Autodesk Inventor part; units mm, degrees
ref_plane "YZ Plane" through (0, 0, 0) normal (1, 0, 0) x (0, 1, 0)
ref_plane "XZ Plane" through (0, 0, 0) normal (0, 1, 0) x (-1, 0, 0)
ref_plane "XY Plane" through (0, 0, 0) normal (0, 0, 1) x (1, 0, 0)
sketch "スケッチ1" plane through (0, 0, 0) normal (0, 0, 1) x (1, 0, 0)
  line L0 (1.55, 2.4) -> (1.55, -2.4)
  line L1 (1.55, -2.4) -> (7, -2.4)
  line L2 (7, -2.4) -> (7, -0.2)
  line L3 (7, -0.2) -> (2, -0.2)
  line L4 (2, -0.2) -> (2, 2.4)
  line L5 (2, 2.4) -> (1.55, 2.4)
  line L6 (0, -3.36) -> (0, 3.36)
  point P0 (0, 0)
  point P1 (1.55, 0)
  dimension "d0" = 1.55
  dimension "d1" = 2
  dimension "d2" = 2.6
  dimension "d3" = 7
  dimension "d4" = 2.2
revolve "回転1" add sketch "スケッチ1" angle 360 about axis through (0, -10, 0) along (0, 1, 0)
sketch "スケッチ2" plane through (0, -0.2, 0) normal (0, 1, 0) x (1, 0, 0)
  circle A0 centre (0, 0) radius 2
  circle A1 centre (0, 0) radius 5.5
  dimension "d6" = 11
extrude "押し出し1" cut sketch "スケッチ2" against normal blind 1
properties part number "足裏_サブフレーム_1_2" material "アセタール樹脂、黒"
Verification items for the finished model (mm, model axes). Give positions to 0.01 mm unless a question says otherwise; leave off trailing zeros. Loops run counter-clockwise (first coordinate to the right, second up) from the corner with the lowest first, then second, coordinate; pieces in that order, holes last. Notation, with made-up numbers: (-23, 3) - (-19, 3) arc R17 cw to (-19, 7) - close; hole circle Ø9 at (-35, 7.25). An arc over 180 degrees is marked (long way). Write item = value, one per line. Start each with the question number.
Q1. Mould release check, pull along Z, two halves, no side actions. Record for faces 1 (the face through (6.466, -1.285, 2.681)), 2 (the face through (0.715, -0.034, -1.375)), 3 (the face through (0, -2.4, -2)): released by +Z, released by -Z, zero draft, split by the parting line, or undercut.
Q2. Cross-section at C-C, the plane y = 1.1. Enter the section's corners in (x, z).
Q3. Cross-section at B-B, the plane z = 0. Enter the section's corners in (x, y), and give its area (3 significant figures).
Q4. Depth check by flat-ended pin: P1, Ø2, axis at y = -0.5, z = 3, coming from the -X side; P2, Ø4, axis at x = 0, z = 0, coming from the -Y side. Enter the tip coordinate at first touch or a pass-through.
Q5. Cross-section at D-D, the plane x = -3. Enter the section's corners in (y, z), and give its area (3 significant figures).
Q6. Cross-section at A-A, the plane x = 0. Enter the section's corners in (y, z).
Q7. Thickness scan on line 1 (Z direction, x = 0, y = -0.8); line 2 (Z direction, x = 0, y = 0.4). Record the ranges inside material, lowest first.
Answer key:
q1.face_1 = split by the parting line
q1.face_2 = undercut
q1.face_3 = zero draft
q2.outline = circle Ø4 at (0, 0); hole circle Ø3.1 at (0, 0)
q3.outline = (-7, -2.4) - (-1.55, -2.4) - (-1.55, 2.4) - (-2, 2.4) - (-2, -1.2) - (-5.5, -1.2) - (-5.5, -0.2) - (-7, -0.2) - close; (1.55, -2.4) - (7, -2.4) - (7, -0.2) - (5.5, -0.2) - (5.5, -1.2) - (2, -1.2) - (2, 2.4) - (1.55, 2.4) - close
q3.area = 19.3 mm^2
q4.P1 = -6.71
q4.P2 = -2.4
q5.outline = (-2.4, -6.32) - (-0.2, -6.32) - (-0.2, -4.61) - (-1.2, -4.61) - (-1.2, 4.61) - (-0.2, 4.61) - (-0.2, 6.32) - (-2.4, 6.32) - close
q5.area = 18.6 mm^2
q6.outline = (-2.4, -7) - (-0.2, -7) - (-0.2, -5.5) - (-1.2, -5.5) - (-1.2, -2) - (2.4, -2) - (2.4, -1.55) - (-2.4, -1.55) - close; (-2.4, 1.55) - (2.4, 1.55) - (2.4, 2) - (-1.2, 2) - (-1.2, 5.5) - (-0.2, 5.5) - (-0.2, 7) - (-2.4, 7) - close
q7.line_1 = -7 to -5.5, -2 to -1.55, 1.55 to 2, 5.5 to 7
q7.line_2 = -2 to -1.55, 1.55 to 2
